Verification items for the finished model (mm, model axes). A direction names the side the tool comes from. Coordinates: 2 decimals unless noted, no trailing zeros. Order: outer loops, then holes, each group sorted by start corner. A loop starts at its lowest first (then second) coordinate and runs counter-clockwise, first axis right, second up.
Q1. Cross-section at B-B, the plane z = -0.75. Count the separate pieces of the cut face and the enclosed holes in it, and give its area (3 significant figures).
Q2. Cross-section at D-D, the plane x = 42. Record the boundary of the cut face in (y, z), and give its area (3 significant figures).
Q3. Set-up check for faces 4 (the flat face through (40, 13, -10.16)), 5 (the cylindrical face through (42.62, 13.92, -5.01)): record each of +Z, -Z, +X, -X, +Y, -Y from which the full face is reachable in a straight line by a thin tool's end or side.
Q4. Cross-section at C-C, the plane x = 25.4. Record the boundary of the cut face in (y, z) (3 decimals).
Q5. Draft check along X on faces 1 (the flat face through (0, 12, 5)), 2 (the cylindrical face through (13.632, 10.768, -5.009)), 3 (the flat face through (50.8, 12, 5)). Enter one of: pulls with the +X half, pulls with the -X half, needs draft (parallel to the pull), parting line crosses it, or undercut.
Q6. Thickness scan on line 1 (X direction, y = 10.5, z = -0.5); line 2 (Z direction, x = 21, y = 22); line 3 (Y direction, x = 26.5, z = -9.5). Record the ranges inside material, lowest first.
Q7. Cross-section at A-A, the plane y = 12.7. Record the boundary of the cut face in (x, z) (1 decimal), and give its area (3 significant figures).
Q8. Depth check by flat-ended pin: P1, Ø4, axis at x = 32.5, y = 12, coming from the -Z side. Enter the tip coordinate at first touch or a pass-through.
from build123d import *

# Parameters (mm, degrees)
F0_W     = 50.8
F0_H     = 25.4
F1_DEPTH = 10.16
F2_R     = 3.175
F3_DEPTH = 10.16
F5_DEPTH = 10.16
F6_DEPTH = 6.35
F7_DEPTH = 6.35


with BuildPart() as f1:
    # F0 (on Top) → F1 (new body)
    with BuildSketch(Plane.XY):
        with Locations((25.4, 12.7)):
            Rectangle(F0_W, F0_H)
    extrude(amount=F1_DEPTH)

    # F2 (on face) → F3 (join)
    with BuildSketch(Plane(origin=(0, 0, 0), x_dir=(1, 0, 0), z_dir=(0, 0, -1))):
        with Locations((25.4, -12.7)):
            Circle(F2_R)
    extrude(amount=F3_DEPTH)

    # F4 (on face) → F5 (join)
    with BuildSketch(Plane(origin=(0, 0, 0), x_dir=(1, 0, 0), z_dir=(0, 0, -1))):
        with BuildLine():
            Line((7.9375, -12.7), (14.2875, -12.7))
            ThreePointArc((14.2875, -12.7), (11.1125, -9.525), (7.9375, -12.7))
        make_face()
        with BuildLine():
            ThreePointArc((7.9375, -12.7), (11.1125, -15.875), (14.2875, -12.7))
            Line((14.2875, -12.7), (7.9375, -12.7))
        make_face()
        with BuildLine():
            Line((42.8625, -12.7), (36.5125, -12.7))
            ThreePointArc((36.5125, -12.7), (39.6875, -15.875), (42.8625, -12.7))
        make_face()
        with BuildLine():
            ThreePointArc((42.8625, -12.7), (39.6875, -9.525), (36.5125, -12.7))
            Line((36.5125, -12.7), (42.8625, -12.7))
        make_face()
    extrude(amount=F5_DEPTH)

    # F6 (add): a face of the model
    f6_faces = [f1.faces().sort_by_distance(p)[0] for p in [
        (25.4, 0, 5.08),
    ]]
    extrude(f6_faces, amount=F6_DEPTH)

    # F7 (add): a face of the model
    f7_faces = [f1.faces().sort_by_distance(p)[0] for p in [
        (25.4, 25.4, 5.08),
    ]]
    extrude(f7_faces, amount=F7_DEPTH)


solid = f1.part
Check values:
1. separate pieces: 3
1. enclosed holes: 0
1. area: 95.0 mm2
2. outline: (-6.35, 0) - (10.52, 0) - (10.52, -10.16) - (14.88, -10.16) - (14.88, 0) - (31.75, 0) - (31.75, 10.16) - (-6.35, 10.16) - close
2. area: 431 mm2
3. face 4: -Z, +X, -X, +Y, -Y
3. face 5: -Z
4. outline: (-6.35, 0) - (9.525, 0) - (9.525, -10.16) - (15.875, -10.16) - (15.875, 0) - (31.75, 0) - (31.75, 10.16) - (-6.35, 10.16) - close
5. face 1: pulls with the -X half
5. face 2: undercut
5. face 3: pulls with the +X half
6. line 1: x = 8.82 to 13.4, 23.11 to 27.69, 37.4 to 41.98
6. line 2: z = 0 to 10.16
6. line 3: y = 9.72 to 15.68
7. outline: (0, 0) - (7.9, 0) - (7.9, -10.2) - (14.3, -10.2) - (14.3, 0) - (22.2, 0) - (22.2, -10.2) - (28.6, -10.2) - (28.6, 0) - (36.5, 0) - (36.5, -10.2) - (42.9, -10.2) - (42.9, 0) - (50.8, 0) - (50.8, 10.2) - (0, 10.2) - close
7. area: 710 mm2
8. P1: stops at z = 0
